Input: part model. Units: mm. Frame: model coordinates. Coordinates: 2 decimals unless noted, no trailing zeros. Write each loop counter-clockwise with the first axis right and the second up, starting at its lowest first coordinate (ties: lowest second). Pieces come first, ordered by that corner, then holes. Notation, with made-up numbers: (19, 74.25) - (39, 74.25) arc R29 cw to (39, 106.25) - close; hole circle Ø2 at (4.5, 15). An arc over 180 degrees is marked (long way). Use a Markdown table: item, result. Add a question column.
Q1. Pin query (flat end, axial travel): P1, Ø10, axis at x = 156.5, y = 62, coming from the -Z side; P2, Ø1, axis at y = 15.5, z = 4.5, coming from the +X side; P3, Ø5, axis at y = 25, z = -4.5, coming from the +X side. Return the tip coordinate at first contact, or that it passes through.
Q2. Material intervals for probe 1 along Y at (x, z) = (65.5, -0.5); probe 2 along X at (y, z) = (85.5, -1); probe 3 along Y at (x, z) = (70.5, 1.5), sorted ascending. Write a range as from..to.
Q3. Section query B-B (y = 13). Return the cut outline in (x, z), then the cut area to 3 significant figures.
Q4. Section query A-A (x = 0). Return the cut outline in (y, z).
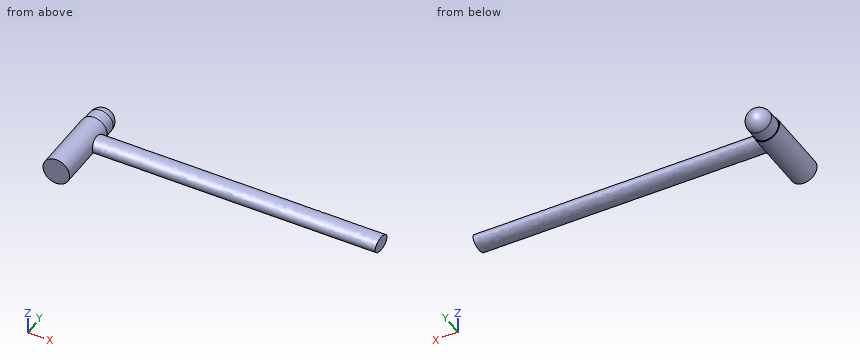
Autodesk Inventor part; units mm, degrees
ref_plane "YZ Plane" through (0, 0, 0) normal (1, 0, 0) x (0, 1, 0)
ref_plane "XZ Plane" through (0, 0, 0) normal (0, 1, 0) x (-1, 0, 0)
ref_plane "XY Plane" through (0, 0, 0) normal (0, 0, 1) x (1, 0, 0)
sketch "Sketch1" plane through (0, 0, 0) normal (0, 1, 0) x (-1, 0, 0)
  circle A0 centre (0, 0) radius 15
  dimension "d0" = 30
extrude "Extrusion1" add sketch "Sketch1" along normal blind 76
sketch "Sketch2" plane through (0, 76, 0) normal (0, 1, 0) x (1, 0, 0)
  circle A0 centre (0, 0) radius 14
  dimension "d3" = 28
extrude "Extrusion2" add sketch "Sketch2" along normal blind 28
fillet "Fillet1" radius 14 1 edges at (-14, 104, 0)
sketch "Sketch3" plane through (0, 0, 0) normal (1, 0, 0) x (0, 1, 0)
  ellipse E0 centre (58, 0) end of major axis (46, 0) minor radius 8
  point P0 (0, 0)
  dimension "d8" = 12
  dimension "d9" = 8
  dimension "d7" = 58
extrude "Extrusion3" add sketch "Sketch3" along normal blind 335
properties part number "Hammer"
Values follow:
| question | item | result |
|---|---|---|
| 1 | P1 | z = -8 |
| 1 | P2 | x = 14.46 |
| 1 | P3 | x = 14.87 |
| 2 | probe 1 | 46.02..69.98 |
| 2 | probe 2 | -13.96..13.96 |
| 2 | probe 3 | 46.21..69.79 |
| 3 | outline | circle Ø30 at (0, 0) |
| 3 | area | 707 mm2 |
| 4 | outline | (0, -15) - (76, -15) - (76, -14) - (90, -14) arc R14 ccw to (90, 14) - (76, 14) - (76, 15) - (0, 15) - close |
